from build123d import *

# Parameters (mm, degrees)
SKETCH1_W                    = 30
SKETCH1_H                    = 60
SKETCH1_R                    = 2
BASE_FLANGE1_DEPTH           = 0.7366
EDGE_FLANGE1_STRIP_W         = 4.4196
EDGE_FLANGE1_STRIP_H         = 0.7366
EDGE_FLANGE1_STRIP_CUT_DEPTH = 30
EDGE_FLANGE1_DEPTH           = 30
EDGE_FLANGE1_PROFILE_W       = 30
EDGE_FLANGE1_PROFILE_H       = 19.2634
EDGE_FLANGE1_PROFILE_R       = 1.625
EDGE_FLANGE1_FLAT_DEPTH      = 0.7366
EDGE_FLANGE6_STRIP_W         = 4.4196
EDGE_FLANGE6_STRIP_H         = 0.7366
EDGE_FLANGE6_STRIP_CUT_DEPTH = 58.5268
EDGE_FLANGE6_DEPTH           = 58.5268
SKETCH24_R                   = 2.05
CUT_EXTRUDE1_DEPTH           = 409.183232337


# Sheet-metal steps are written as plain solids
with BuildPart() as part:
    # Sketch1 → Base-Flange1 (new body)
    with BuildSketch(Plane(origin=(0, 0, 0), x_dir=(1, 0, 0), z_dir=(0, 1, 0))):
        Rectangle(SKETCH1_W, SKETCH1_H)
        with Locations(Location((7.5, -15, 0), (0, 0, 270))):
            Circle(SKETCH1_R, mode=Mode.SUBTRACT)
        with Locations(Location((0, 15, 0), (0, 0, 270))):
            Circle(SKETCH1_R, mode=Mode.SUBTRACT)
        with Locations(Location((-7.5, -15, 0), (0, 0, 270))):
            Circle(SKETCH1_R, mode=Mode.SUBTRACT)
    extrude(amount=-BASE_FLANGE1_DEPTH)

    # Edge-Flange1 strip (across the edge) → Edge-Flange1 strip cut (cut)
    with BuildSketch(Plane(origin=(15, 0, -30), x_dir=(0, 0, 1), z_dir=(-1, 0, 0))):
        with Locations((-0.7366, -0.3683)):
            Rectangle(EDGE_FLANGE1_STRIP_W, EDGE_FLANGE1_STRIP_H)
    extrude(amount=EDGE_FLANGE1_STRIP_CUT_DEPTH, mode=Mode.SUBTRACT)

    # Edge-Flange1 bend section (across the edge) → Edge-Flange1 (add)
    with BuildSketch(Plane(origin=(15, 0, -30), x_dir=(0, 0, 1), z_dir=(-1, 0, 0))):
        with BuildLine():
            Line((0, 0.7366), (0.7366, 0.7366))
            ThreePointArc((0.7366, 0.7366), (0.952345145, 0.215745145), (1.4732, 0))
            Line((1.4732, 0), (1.4732, -0.7366))
            ThreePointArc((1.4732, -0.7366), (0.43149029, -0.30510971), (0, 0.7366))
        make_face()
    extrude(amount=EDGE_FLANGE1_DEPTH)

    # Edge-Flange1 profile (on flange) → Edge-Flange1 flat (add)
    with BuildSketch(Plane(origin=(0, 0, -30), x_dir=(-1, 0, 0), z_dir=(0, 0, -1))):
        with Locations((0, 10.3683)):
            Rectangle(EDGE_FLANGE1_PROFILE_W, EDGE_FLANGE1_PROFILE_H)
        with Locations((0, 10)):
            Circle(EDGE_FLANGE1_PROFILE_R, mode=Mode.SUBTRACT)
    extrude(amount=-EDGE_FLANGE1_FLAT_DEPTH)

    # Edge-Flange6 strip (across the edge) → Edge-Flange6 strip cut (cut)
    with BuildSketch(Plane(origin=(15, 0, 30), x_dir=(-1, 0, 0), z_dir=(0, 0, -1))):
        with Locations((-1.4732, -0.3683)):
            Rectangle(EDGE_FLANGE6_STRIP_W, EDGE_FLANGE6_STRIP_H)
    extrude(amount=EDGE_FLANGE6_STRIP_CUT_DEPTH, mode=Mode.SUBTRACT)

    # Edge-Flange6 section (across the edge) → Edge-Flange6 (add)
    with BuildSketch(Plane(origin=(15, 0, 30), x_dir=(-1, 0, 0), z_dir=(0, 0, -1))):
        with BuildLine():
            Line((-0.7366, 0.7366), (-0.7366, 19.2634))
            Line((-0.7366, 19.2634), (0, 19.2634))
            Line((0, 19.2634), (0, 0.7366))
            ThreePointArc((0, 0.7366), (0.215745145, 0.215745145), (0.7366, 0))
            Line((0.7366, 0), (0.7366, -0.7366))
            ThreePointArc((0.7366, -0.7366), (-0.30510971, -0.30510971), (-0.7366, 0.7366))
        make_face()
    extrude(amount=EDGE_FLANGE6_DEPTH)

    # Sketch24 → Cut-Extrude1 (cut, through all)
    with BuildSketch(Plane(origin=(385, -11.740421973, -44.873872437), x_dir=(0, 0, -1), z_dir=(1, 0, 0))):
        with Locations((-42.610472437, 21.740421973)):
            Circle(SKETCH24_R)
        with Locations((-58.610472437, 21.740421973)):
            Circle(SKETCH24_R)
    extrude(amount=-CUT_EXTRUDE1_DEPTH, mode=Mode.SUBTRACT)


solid = part.part
Could you check a few things on this model? Use its own coordinates, in mm. A direction names the side the tool comes from. Round coordinates to 2 decimals unless told otherwise and drop trailing zeros. Write each loop counter-clockwise with the first axis right and the second up, starting at its lowest first coordinate (ties: lowest second). Pieces come first, ordered by that corner, then holes. Notation, with made-up numbers: (0.5, 59) -> (26.5, 59) arc R15 ccw to (26.5, 85) -> close; hole circle Ø10 at (21, -31). An arc over 180 degrees is marked (long way). Use a Markdown table: item, result.
1. If we section it at D-D (x = 0): List the corners of the cut face in (y, z) for me (3 decimals).
Answer key:
| item | result |
|---|---|
| outline | (-0.737, -28.527) arc R1.473 ccw to (0.737, -30) -> (8.375, -30) -> (8.375, -29.263) -> (0.737, -29.263) arc R0.737 cw to (0, -28.527) -> (0, -17) -> (-0.737, -17) -> close; (-0.737, -13) -> (0, -13) -> (0, 30) -> (-0.737, 30) -> close; (11.625, -30) -> (20, -30) -> (20, -29.263) -> (11.625, -29.263) -> close |
2. We'd pull the mould along X, two halves only. Please class faces 1 (the face through (15.37, 8, -1.82)), 2 (the face through (-15, -0.4, -0.1)), 3 (the face through (0.352, 8.414, -29.637)), 4 (the face through (15, 9.5, -29.6)): +X half, -X half, draft (parallel to the pull), parting line (faces both ways), or undercut.
Answer key:
| item | result |
|---|---|
| face 1 | draft |
| face 2 | -X half |
| face 3 | undercut |
| face 4 | +X half |
3. Which directions (+Z, -Z, +X, -X, +Y, -Y) give clear straight access to the entire face, cutting with the end or side of a thin tool? Please do faces 5 (the face through (0, 13, -29.263)), 6 (the face through (15.29, -0.32, 1.15)), 7 (the face through (15, 10, 1)).
Answer key:
| item | result |
|---|---|
| face 5 | +Z, +X, -X, +Y |
| face 6 | +Z, +X, -Y |
| face 7 | +Z, -X, +Y |
4. Please list where these lines run through material, in increasing order: probe 1 along Z at (x, y) = (9.5, 8); probe 2 along X at (y, z) = (-0.2, 15); probe 3 along X at (y, z) = (18.25, 13).
Answer key:
| item | result |
|---|---|
| probe 1 | z = -30 to -29.26 |
| probe 2 | x = -15 to -9.5, -5.5 to 5.5, 9.5 to 15.4 |
| probe 3 | x = 15 to 15.74 |
5. If we section it at C-C (y = 10): List the corners of the cut face in (x, z) for me (3 decimals).
Answer key:
| item | result |
|---|---|
| outline | (-15, -30) -> (-1.625, -30) -> (-1.625, -29.263) -> (-15, -29.263) -> close; (1.625, -30) -> (15, -30) -> (15, -29.263) -> (1.625, -29.263) -> close; (15, -28.527) -> (15.737, -28.527) -> (15.737, -4.313) -> (15, -4.313) -> close; (15, -0.213) -> (15.737, -0.213) -> (15.737, 11.687) -> (15, 11.687) -> close; (15, 15.787) -> (15.737, 15.787) -> (15.737, 30) -> (15, 30) -> close |
6. If we section it at B-B (x = 7.5): List the corners of the cut face in (y, z) for me.
Answer key:
| item | result |
|---|---|
| outline | (-0.74, -28.53) arc R1.47 ccw to (0.74, -30) -> (20, -30) -> (20, -29.26) -> (0.74, -29.26) arc R0.74 cw to (0, -28.53) -> (0, 13) -> (-0.74, 13) -> close; (-0.74, 17) -> (0, 17) -> (0, 30) -> (-0.74, 30) -> close |
7. For pin 1 Ø1.6 at (y, z) = (11.5, -29.5) entering from +X; pin 2 Ø4 at (x, y) = (0, 10) entering from +Z; pin 3 Ø6 at (x, z) = (-1, -17) entering from +Y; pin 4 Ø2.5 at (y, z) = (10, 13.74) entering from +X (3 decimals), each with a flat end and sliding along its axis, tell me the tip position at first contact or that it passes through.
Answer key:
| item | result |
|---|---|
| pin 1 | stops at x = 15 |
| pin 2 | stops at z = -29.26 |
| pin 3 | stops at y = 0 |
| pin 4 | passes through |
8. If we section it at A-A (z = -15): List the corners of the cut face in (x, y) for me.
Answer key:
| item | result |
|---|---|
| outline | (-15, -0.74) -> (-2, -0.74) -> (-2, 0) -> (-15, 0) -> close; (2, -0.74) -> (14.26, -0.74) arc R1.47 ccw to (15.74, 0.74) -> (15.74, 19.26) -> (15, 19.26) -> (15, 0.74) arc R0.74 cw to (14.26, 0) -> (2, 0) -> close |
